The drawing under review shows one solid part. Ordinate dimensions are in mm from its lowest x, y, z. A direction names the side the tool comes from. Round coordinates to 2 decimals unless told otherwise and drop trailing zeros. Loops run counter-clockwise (first coordinate to the right, second up) from the corner with the lowest first, then second, coordinate; pieces in that order, holes last. Notation, with made-up numbers: M -27.5,57.5 L -22.5,57.5 A16 cw -22.5,66.5 Z; hole C 21.25,32.5 d2. An arc over 180 degrees is marked long. Use a Markdown table: item, result.
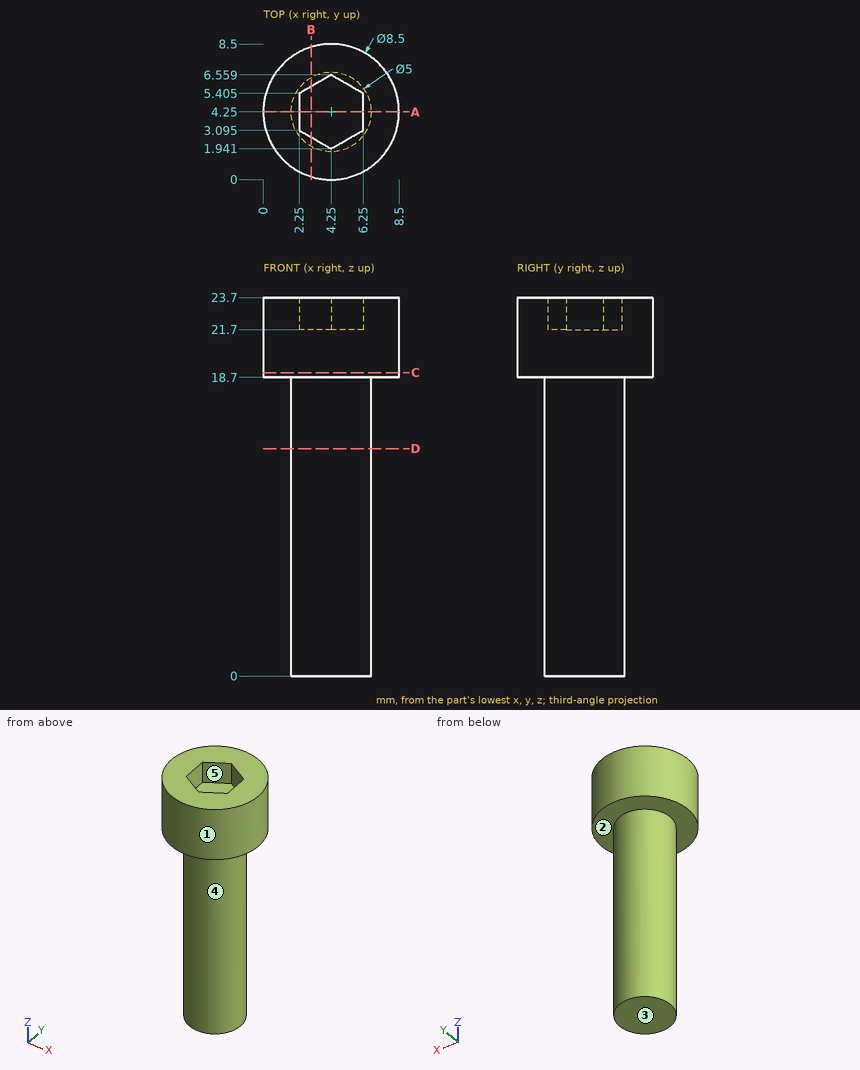
1. Take a section at A-A on y = 4.25. Give the boundary of the cut face in (x, z), and give its area (3 significant figures).
Check values:
| item | result |
|---|---|
| outline | M 0,18.7 L 1.75,18.7 L 1.75,0 L 6.75,0 L 6.75,18.7 L 8.5,18.7 L 8.5,23.7 L 6.25,23.7 L 6.25,21.7 L 2.25,21.7 L 2.25,23.7 L 0,23.7 Z |
| area | 128 mm² |
2. Take a section at C-C on z = 19. Give the boundary of the cut face in (x, y).
Check values:
| item | result |
|---|---|
| outline | C 4.25,4.25 d8.5 |
3. Insertion check: pin 1 (1.5 mm diameter, centred on x = 1.5, y = 5.5, fed in from -Z); pin 2 (1 mm diameter, centred on y = 5, z = 3.5, fed in from -X). Each pin has a flat end and moves straight along its axis. Give the tip position at first contact, or say it passes through.
Check values:
| item | result |
|---|---|
| pin 1 | stops at z = 0 |
| pin 2 | stops at x = 1.76 |
4. Machinability: for the marked faces 1 and 2, which of the approach directions +Z, -Z, +X, -X, +Y, -Y give a long, thin tool a straight path to every point of the face, cutting with its end or side? Answer none if there is none.
Check values:
| item | result |
|---|---|
| face 1 | +Z, -Z |
| face 2 | -Z |
5. Take a section at D-D on z = 14.25. Give the boundary of the cut face in (x, y), and give its area (3 significant figures).
Check values:
| item | result |
|---|---|
| outline | C 4.25,4.25 d5 |
| area | 19.6 mm² |
6. The part is to be moulded in two halves that separate along Y. For the marked faces 3, 4 and 5, say which applies: pulls with the +Y half, pulls with the -Y half, needs draft (parallel to the pull), parting line crosses it, or undercut.
Check values:
| item | result |
|---|---|
| face 3 | needs draft |
| face 4 | parting line crosses it |
| face 5 | undercut |
7. Wall thickness on line 1 along Z through (x, y) = (7.25, 3.5); line 2 along Z through (x, y) = (4.5, 3.75); line 3 along Y through (x, z) = (2.75, 22) (1 decimal): over which ranges is each line inside the solid? List them lowest first. Write a range as from..to.
Check values:
| item | result |
|---|---|
| line 1 | z = 18.7..23.7 |
| line 2 | z = 0..21.7 |
| line 3 | y = 0.3..2.8, 5.7..8.2 |
8. Take a section at B-B on x = 3. Give the boundary of the cut face in (y, z) (1 decimal), and give its area (3 significant figures).
Check values:
| item | result |
|---|---|
| outline | M 0.2,18.7 L 2.1,18.7 L 2.1,0 L 6.4,0 L 6.4,18.7 L 8.3,18.7 L 8.3,23.7 L 5.8,23.7 L 5.8,21.7 L 2.7,21.7 L 2.7,23.7 L 0.2,23.7 Z |
| area | 115 mm² |
